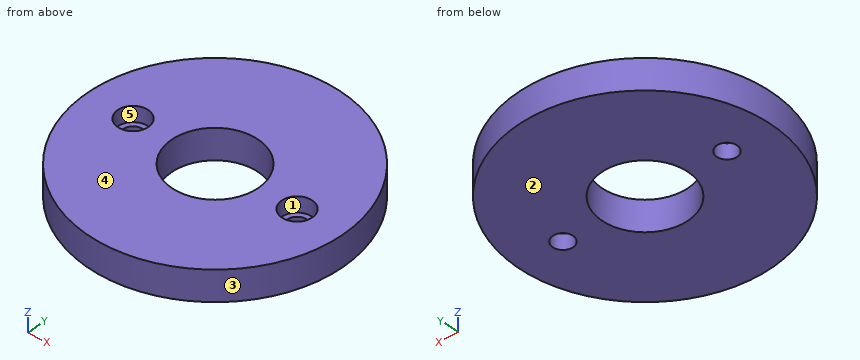
```python
from build123d import *

# Parameters (mm, degrees)
ESQUISSE1_R             = 25
ESQUISSE1_R_2           = 8.5
BOSS_EXTRU_3_DEPTH      = 6
ESQUISSE6_R             = 3
ENL_V_MAT_EXTRU_7_DEPTH = 3
ESQUISSE7_R             = 2
ENL_V_MAT_EXTRU_8_DEPTH = 91


with BuildPart() as part:
    # Esquisse1 → Boss.-Extru.3 (new body)
    with BuildSketch(Plane.XY):
        Circle(ESQUISSE1_R)
        Circle(ESQUISSE1_R_2, mode=Mode.SUBTRACT)
    extrude(amount=BOSS_EXTRU_3_DEPTH)

    # Esquisse6 → Enlèv. mat.-Extru.7 (cut)
    with BuildSketch(Plane.XY.offset(6)):
        with Locations((-16, 0)):
            Circle(ESQUISSE6_R)
        with Locations(Location((16, 0, 0), (0, 0, 180))):
            Circle(ESQUISSE6_R)
    extrude(amount=-ENL_V_MAT_EXTRU_7_DEPTH, mode=Mode.SUBTRACT)

    # Esquisse7 → Enlèv. mat.-Extru.8 (cut)
    with BuildSketch(Plane.XY.offset(6)):
        with Locations((-16, 0)):
            Circle(ESQUISSE7_R)
        with Locations((16, 0)):
            Circle(ESQUISSE7_R)
    extrude(amount=-ENL_V_MAT_EXTRU_8_DEPTH, mode=Mode.SUBTRACT)


solid = part.part
```
CAD build for the part. Positions are in the model's coordinates, mm. Face numbers are marked on the shaded views. A direction names the side the tool comes from. Round coordinates to 2 decimals unless told otherwise and drop trailing zeros. Loops run counter-clockwise (first coordinate to the right, second up) from the corner with the lowest first, then second, coordinate; pieces in that order, holes last. Notation, with made-up numbers: M 15,-23 L 59,-23 A33 cw 59,14 Z; hole C -4.5,-14 d4. An arc over 180 degrees is marked long. Use a Markdown table: item, result. Add a question column.
(1) Flat gauge pins, fed straight in: pin 1 (1.5 mm diameter, centred on y = 14, z = 2, fed in from +X); pin 2 (1.5 mm diameter, centred on x = -0.5, z = 1.5, fed in from -Y); pin 3 (2 mm diameter, centred on x = -17, z = 2.5, fed in from +Y). Where does each tip first touch, or does it go through?
(2) Cut at B-B (y = 0). Give the cut face in (x, z), and give its area (3 significant figures).
(3) Pull direction Y, two halves, no side cores. Call the marked faces 1, 2 and 3: +Y half, -Y half, draft (parallel to the pull), parting line (faces both ways), or undercut.
(4) Cut at A-A (x = -3.5). Give the cut face in (y, z).
(5) Cut at C-C (z = 1.95). Give the cut face in (x, y), and give its area (3 significant figures).
(6) Cut at D-D (x = -16). Give the cut face in (y, z).
(7) Which spindle directions (+Z, -Z, +X, -X, +Y, -Y) get a long thin tool onto all of the face, cutting with end or side? Do the marked faces 4 and 5. Say none if no direction does.
(8) Drill centre lines: line 1 (Y direction, x = 0, z = 2.9); line 2 (Y direction, x = -16, z = 1.8); line 3 (Y direction, x = -19.5, z = 4.75). Where is each one in solid material? Low to high.
Geometry says:
| question | item | result |
|---|---|---|
| 1 | pin 1 | stops at x = 21.2 |
| 1 | pin 2 | stops at y = -25 |
| 1 | pin 3 | stops at y = 19.21 |
| 2 | outline | M -25,0 L -18,0 L -18,3 L -19,3 L -19,6 L -25,6 Z; M -14,0 L -8.5,0 L -8.5,6 L -13,6 L -13,3 L -14,3 Z; M 8.5,0 L 14,0 L 14,3 L 13,3 L 13,6 L 8.5,6 Z; M 18,0 L 25,0 L 25,6 L 19,6 L 19,3 L 18,3 Z |
| 2 | area | 138 mm² |
| 3 | face 1 | undercut |
| 3 | face 2 | draft |
| 3 | face 3 | parting line |
| 4 | outline | M -24.75,0 L -7.75,0 L -7.75,6 L -24.75,6 Z; M 7.75,0 L 24.75,0 L 24.75,6 L 7.75,6 Z |
| 5 | outline | C 0,0 d50; hole C -16,0 d4; hole C 0,0 d17; hole C 16,0 d4 |
| 5 | area | 1,710 mm² |
| 6 | outline | M -19.21,0 L -2,0 L -2,3 L -3,3 L -3,6 L -19.21,6 Z; M 2,0 L 19.21,0 L 19.21,6 L 3,6 L 3,3 L 2,3 Z |
| 7 | face 4 | +Z, +X, -X, +Y, -Y |
| 7 | face 5 | +Z |
| 8 | line 1 | y = -25 to -8.5, 8.5 to 25 |
| 8 | line 2 | y = -19.21 to -2, 2 to 19.21 |
| 8 | line 3 | y = -15.64 to 15.64 |
